Autodesk Inventor part; units mm, degrees
ref_plane "YZ Plane" through (0, 0, 0) normal (1, 0, 0) x (0, 1, 0)
ref_plane "XZ Plane" through (0, 0, 0) normal (0, 1, 0) x (-1, 0, 0)
ref_plane "XY Plane" through (0, 0, 0) normal (0, 0, 1) x (1, 0, 0)
sketch "Sketch1" plane through (0, 0, 0) normal (0, 0, 1) x (1, 0, 0)
  line L0 (40, 20.5) -> (40, -20.5)
  line L1 (-40, 20.5) -> (40, 20.5)
  line L2 (-40, -20.5) -> (-40, 20.5)
  line L3 (40, -20.5) -> (-40, -20.5)
  line L4 (40, 20.5) -> (40, -20.5)
  line L5 (40, -20.5) -> (-40, -20.5)
  line L6 (-40, -20.5) -> (-40, 20.5)
  line L7 (-40, 20.5) -> (40, 20.5)
  line L8 (37, 23.5) -> (-37, 23.5)
  line L9 (-43, 17.5) -> (-43, -17.5)
  line L10 (-37, -23.5) -> (37, -23.5)
  line L11 (43, -17.5) -> (43, 17.5)
  line L12 (34.23, -11.25) -> (34.23, 10.75)
  line L13 (5.23, -11.25) -> (34.23, -11.25)
  line L14 (5.23, 10.75) -> (5.23, -11.25)
  line L15 (34.23, 10.75) -> (5.23, 10.75)
  circle A0 centre (-26.5, 0.5) radius 5
  arc A1 (37, -23.5) -> (43, -17.5) centre (37, -17.5) ccw
  arc A2 (43, 17.5) -> (37, 23.5) centre (37, 17.5) ccw
  arc A3 (-37, 23.5) -> (-43, 17.5) centre (-37, 17.5) ccw
  arc A4 (-43, -17.5) -> (-37, -23.5) centre (-37, -17.5) ccw
  point P0 (0, 0)
extrude "Extrusion1" add sketch "Sketch1" along normal blind 3 contours L0 L3 L2 L1 | A2 L11 A1 L10 A4 L9 A3 L8 | L13 L14 L15 L12 | A0
sketch "Sketch2" plane through (0, 0, 3) normal (0, 0, 1) x (1, 0, 0)
  line L0 (39.5, 20) -> (-39.5, 20)
  line L1 (-39.5, 20) -> (-39.5, -20)
  line L2 (-39.5, -20) -> (39.5, -20)
  line L3 (39.5, -20) -> (39.5, 20)
  line L4 (-17.5, 15.5) -> (-1.5, 15.5)
  line L5 (-1.5, 15.5) -> (-1.5, -2)
  line L6 (-1.5, -2) -> (-17.5, -2)
  line L7 (-17.5, -2) -> (-17.5, 15.5)
  line L8 (-17.5, 15.5) -> (-1.5, -2) construction
  line L9 (-1.5, 15.5) -> (-17.5, -2) construction
  point P0 (0, 0)
  point P1 (-9.5, 6.75)
  dimension "d2" = 16
  dimension "d3" = 17.5
  dimension "d4" = 18
  dimension "d6" = 41
extrude "Extrusion2" cut sketch "Sketch2" against normal blind 3 contours L4 L5 L6 L7
chamfer "Chamfer1" distance 2 angle 45 4 edges at (-1.5, 6.75, 3) (-17.5, 6.75, 3) (-9.5, -2, 3) (-9.5, 15.5, 3)
sketch "Sketch3" plane through (0, 0, 3) normal (0, 0, 1) x (1, 0, 0)
  line L0 (37, 23.5) -> (-37, 23.5)
  arc A0 (-37, 23.5) -> (-43, 17.5) centre (-37, 17.5) ccw
  line L1 (-43, 17.5) -> (-43, -17.5)
  arc A1 (-43, -17.5) -> (-37, -23.5) centre (-37, -17.5) ccw
  line L2 (-37, -23.5) -> (37, -23.5)
  arc A2 (37, -23.5) -> (43, -17.5) centre (37, -17.5) ccw
  line L3 (43, -17.5) -> (43, 17.5)
  arc A3 (43, 17.5) -> (37, 23.5) centre (37, 17.5) ccw
  line L4 (34.23, -11.25) -> (34.23, 10.75)
  line L5 (5.23, -11.25) -> (34.23, -11.25)
  line L6 (5.23, 10.75) -> (5.23, -11.25)
  line L7 (34.23, 10.75) -> (5.23, 10.75)
  line L8 (40, 20.5) -> (40, -20.5)
  line L9 (-40, 20.5) -> (40, 20.5)
  line L10 (-40, -20.5) -> (-40, 20.5)
  line L11 (40, -20.5) -> (-40, -20.5)
  circle A4 centre (-26.5, 0.5) radius 5
  point P0 (0, 0)
extrude "Extrusion3" cut sketch "Sketch3" against normal blind 3 contours A3 L3 A2 L2 A1 L1 A0 L0
sketch "Sketch4" plane through (0, 0, 3) normal (0, 0, 1) x (1, 0, 0)
  line L0 (40, 20.5) -> (-40, 20.5)
  line L1 (-40, 20.5) -> (-40, -20.5)
  line L2 (-40, -20.5) -> (40, -20.5)
  line L3 (40, -20.5) -> (40, 20.5)
  line L4 (-39.25, 19.75) -> (39.25, 19.75)
  line L5 (39.25, 19.75) -> (39.25, -19.75)
  line L6 (39.25, -19.75) -> (-39.25, -19.75)
  line L7 (-39.25, -19.75) -> (-39.25, 19.75)
  line L8 (-39.25, 19.75) -> (39.25, -19.75) construction
  line L9 (39.25, 19.75) -> (-39.25, -19.75) construction
  point P0 (0, 0)
  dimension "d14" = 78.5
  dimension "d15" = 39.5
extrude "Extrusion4" cut sketch "Sketch4" against normal blind 3
sketch "Sketch5" plane through (0, 0, 0) normal (0, 0, -1) x (-1, 0, 0)
  line L0 (39.25, -19.75) -> (39.25, 19.75)
  line L1 (39.25, 19.75) -> (-39.25, 19.75)
  line L2 (-39.25, 19.75) -> (-39.25, -19.75)
  line L3 (-39.25, -19.75) -> (39.25, -19.75)
  line L4 (17.5, 15.5) -> (17.5, -2)
  line L5 (17.5, -2) -> (1.5, -2)
  line L6 (1.5, -2) -> (1.5, 15.5)
  line L7 (1.5, 15.5) -> (17.5, 15.5)
  point P0 (0, 0)
sketch "Sketch6" plane through (39.25, -19.75, 3) normal (1, 0, 0) x (0, 0, -1)
  line L0 (3, 39.5) -> (3, 0)
  line L1 (3, 30.3376) -> (7.1898, 28.4353) construction
  line L2 (7.1898, 28.4353) -> (10.8762, 26.1607) construction
  line L3 (10.8762, 26.1607) -> (12.9155, 21.0624) construction
  line L4 (12.9155, 21.0624) -> (12.9155, 15.718) construction
  line L5 (12.9155, 15.718) -> (7.6212, 12.5523) construction
  line L6 (7.6212, 12.5523) -> (3, 10.7087) construction
  spline S0 degree 4 poles (3, 30.3376) (7.1898, 28.4353) (10.8762, 26.1607) (12.9155, 21.0624) (12.9155, 15.718) (7.6212, 12.5523) (3, 10.7087) knots 1 1 1 1 1 2 3 4 4 4 4 4
  line L7 (3, 30.3376) -> (3, 10.7087)
  point P0 (3, 19.75)
extrude "Extrusion5" add sketch "Sketch6" against normal blind 3
sketch "Sketch7" plane through (-39.25, -19.75, 3) normal (-1, 0, 0) x (0, 0, 1)
  line L0 (-3, 30.3376) -> (-3, 10.7087)
  spline S0 degree 4 poles (-3, 30.3376) (-7.1898, 28.4353) (-10.8762, 26.1607) (-12.9155, 21.0624) (-12.9155, 15.718) (-7.6212, 12.5523) (-3, 10.7087) knots 0 0 0 0 0 0.333333 0.666667 1 1 1 1 1
  point P0 (-3, 19.75)
extrude "Extrusion6" add sketch "Sketch7" against normal blind 3
sketch "Sketch8" plane through (39.25, -19.75, 3) normal (1, 0, 0) x (0, 0, -1)
  line L0 (0, 0) -> (0, 39.5)
  circle A0 centre (10, 19.75) radius 1.2
  point P0 (3, 19.75)
  dimension "d22" = 2.4
  dimension "d23" = 10
extrude "Extrusion7" cut sketch "Sketch8" against normal through all
chamfer "Chamfer2" distance 0.5 angle 45 2 edges at (39.25, 0, -5.8) (-39.25, 0, -5.8)
sketch "Sketch9" plane through (0, 0, 0) normal (0, 0, -1) x (-1, 0, 0)
  line L0 (39.25, -9.0413) -> (36.25, -9.0413)
  line L1 (36.25, -9.0413) -> (36.25, 10.5876)
  line L2 (36.25, 10.5876) -> (39.25, 10.5876)
  line L3 (39.25, 10.5876) -> (39.25, 19.75)
  line L4 (39.25, 19.75) -> (-39.25, 19.75)
  line L5 (-39.25, 19.75) -> (-39.25, 10.5876)
  line L6 (-39.25, 10.5876) -> (-36.25, 10.5876)
  line L7 (-36.25, 10.5876) -> (-36.25, -9.0413)
  line L8 (-36.25, -9.0413) -> (-39.25, -9.0413)
  line L9 (-39.25, -9.0413) -> (-39.25, -19.75)
  line L10 (-39.25, -19.75) -> (39.25, -19.75)
  line L11 (39.25, -19.75) -> (39.25, -9.0413)
  line L12 (17.5, 15.5) -> (17.5, -2)
  line L13 (17.5, -2) -> (1.5, -2)
  line L14 (1.5, -2) -> (1.5, 15.5)
  line L15 (1.5, 15.5) -> (17.5, 15.5)
  point P0 (0, 0)
properties part number "obudowa - timer- back"
Source: CAD feature listing. Evaluate the final solid. Frame: model axes, mm. A direction names the side the tool comes from. Give positions to 0.01 mm unless a question says otherwise; leave off trailing zeros. Write each loop counter-clockwise with the first axis right and the second up, starting at its lowest first coordinate (ties: lowest second). Pieces come first, ordered by that corner, then holes. Notation, with made-up numbers: (-6.5, -18.5) - (46.5, -18.5) arc R13 cw to (46.5, 0.5) - close; hole circle Ø2 at (88, -25.5). An arc over 180 degrees is marked (long way). Write item = value, one per line. Start each with the question number.
Q1. Material intervals for probe 1 along X at (y, z) = (7.5, -2); probe 2 along Z at (x, y) = (28.5, -3); probe 3 along Y at (x, z) = (38.1, -7), sorted ascending.
Q2. Draft query along X for faces 4 (the flat face through (-39.25, 0, 0)), 5 (the flat face through (-9.6, 16.5, 2)), 6 (the flat face through (-1, 19.75, 2)). Return one class per face: +X half, -X half, draft (parallel to the pull), parting line (faces both ways), or undercut.
Q3. Cut plane A-A, the plane x = -10. Return loops of the section in (y, z).
Q4. Cut plane D-D, the plane x = 29. Return loops of the section in (y, z), then the cut area to 4 significant figures.
Q5. Pin query (flat end, axial travel): pin 1 Ø3 at (y, z) = (0, -7) entering from +X; pin 2 Ø1 at (x, y) = (-31, -15) entering from -Z; pin 3 Ø1.9 at (y, z) = (0, -7) entering from -X. Return the tip coordinate at first contact, or that it passes through.
Q6. Reachability of faces 1 (the cylindrical face through (-37.48, 0.05, -5.8)), 2 (the flat face through (-36.25, 1, -4)), 3 (the flat face through (-9, -3, 2)) from +Z, -Z, +X, -X, +Y, -Y: full face, straight path, thin tool, end or side. Return the list, or none.
Q7. Cut plane B-B, the plane y = 0. Give the number of separate pieces and of enclosed holes in the cut face, then the cut area to 3 significant figures.
Computed values:
q1.probe_1 = -39.25 to -36.25, 36.25 to 39.25
q1.probe_2 = 0 to 3
q1.probe_3 = -5.26 to -1.2, 1.2 to 6.21
q2.face_4 = -X half
q2.face_5 = undercut
q2.face_6 = draft
q3.outline = (-19.75, 0) - (-2, 0) - (-2, 1) - (-4, 3) - (-19.75, 3) - close; (15.5, 0) - (19.75, 0) - (19.75, 3) - (17.5, 3) - (15.5, 1) - close
q4.outline = (-19.75, 0) - (19.75, 0) - (19.75, 3) - (-19.75, 3) - close
q4.area = 118.5 mm²
q5.pin_1 = 39.05
q5.pin_2 = 0
q5.pin_3 = through
q6.face_1 = +X, -X
q6.face_2 = -Z, +Y, -Y
q6.face_3 = +Z
q7.separate_pieces = 4
q7.enclosed_holes = 0
q7.area = 225 mm²
